Check sheet for the drawn part. Datum: minimum x, y, z corner. Units: mm. A direction names the side the tool comes from. Coordinates: 2 decimals unless noted, no trailing zeros. Order: outer loops, then holes, each group sorted by start corner. A loop starts at its lowest first (then second) coordinate and runs counter-clockwise, first axis right, second up. Notation, with made-up numbers: (-3.75, -10.5) - (9.25, -10.5) arc R32 cw to (9.25, 18.5) - close; hole circle Ø4 at (33.5, -22.5). An arc over 180 degrees is marked (long way). Return JSON: item names as keys, results as strings. Group by question number.
Item 1: Tool access check on the marked faces 1 and 2. Record the directions out of +Z, -Z, +X, -X, +Y, -Y that give a thin tool (end or side, any length) a straight path to the whole face; none if there is none.
Item 2: Section check D-D on z = 7.5. Enter the section's corners in (x, y).
Item 3: Scan lines: probe 1 along Y at (x, z) = (25.4, 57.25); probe 2 along Z at (x, y) = (4.75, 12.7) (3 decimals); probe 3 along Y at (x, z) = (5.5, 13.5). Record each from-to range of solid material in increasing order.
Item 4: Gauge pin test, flat ends, axial feed: pin 1 (4 mm diameter, centred on y = 76.2, z = 12.7, fed in from -X); pin 2 (5 mm diameter, centred on x = 10.5, y = 11.5, fed in from -Z) (3 decimals); pin 3 (1.5 mm diameter, centred on y = 78.5, z = 52.5, fed in from +X); pin 4 (6 mm diameter, centred on y = 10.5, z = 36.5, fed in from +X). Record the tip position at first contact, or that the pin passes through.
Item 5: Section check A-A on x = 25.4. Give the number of separate pieces and of enclosed holes in the cut face, then the cut area to 3 significant figures.
Item 6: Section check B-B on y = 55. Enter the section's corners in (x, z) (3 decimals), then the cut area to 3 significant figures.
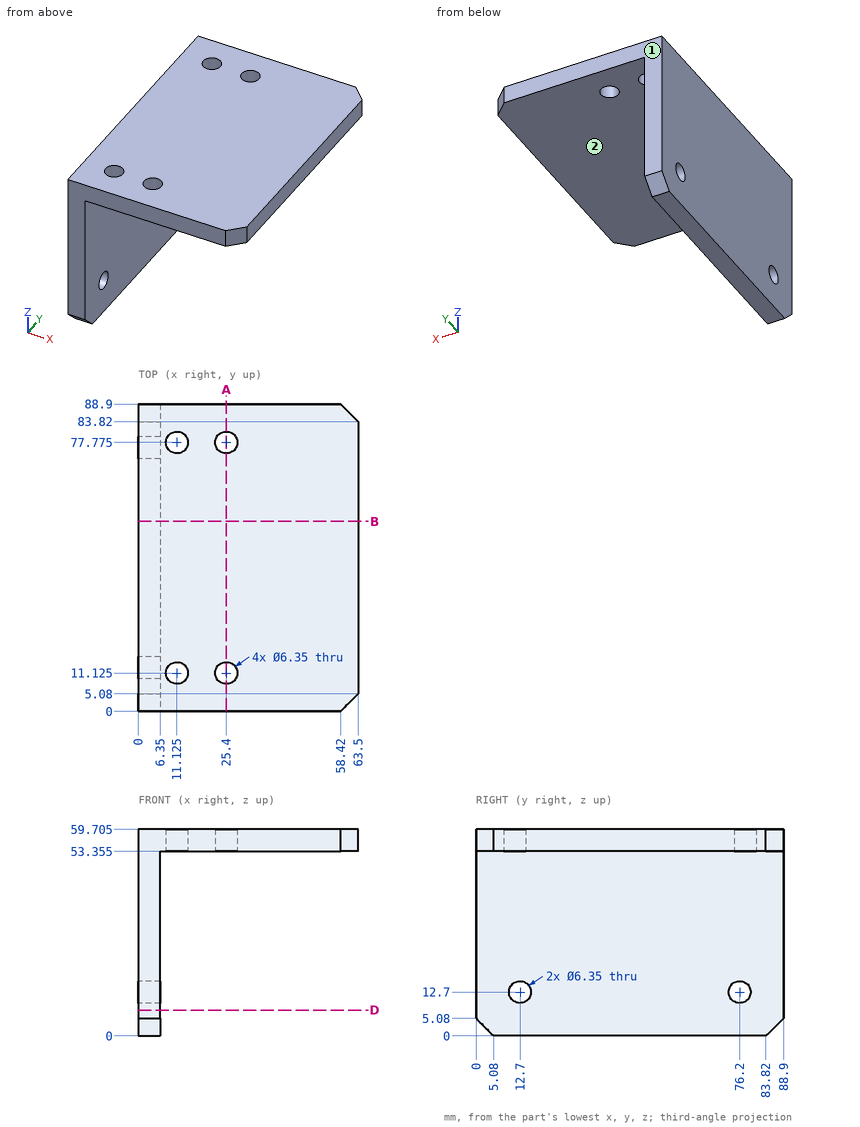
Computed:
{
 "1": {"face 1": "+Z, -Z, +X, -X, +Y", "face 2": "-Z, +X, +Y, -Y"},
 "2": {"outline": "(0, 0) - (6.35, 0) - (6.35, 88.9) - (0, 88.9) - close"},
 "3": {"probe 1": "y = 0 to 7.95, 14.3 to 74.6, 80.95 to 88.9", "probe 2": "z = 0 to 9.525, 15.875 to 59.705", "probe 3": "y = 0 to 9.63, 15.77 to 73.13, 79.27 to 88.9"},
 "4": {"pin 1": "passes through", "pin 2": "stops at z = 53.355", "pin 3": "stops at x = 6.35", "pin 4": "stops at x = 6.35"},
 "5": {"separate pieces": "3", "enclosed holes": "0", "area": "484 mm²"},
 "6": {"outline": "(0, 0) - (6.35, 0) - (6.35, 53.355) - (63.5, 53.355) - (63.5, 59.705) - (0, 59.705) - close", "area": "742 mm²"}
}
